```python
from build123d import *

# Parameters (mm, degrees)
SKETCH018_R          = 70
PAD010_DEPTH         = 7
SKETCH019_R          = 2.5
POCKET_DEPTH         = 3.5
POLARPATTERN_COUNT   = 4
SKETCH_R             = 7.5
SKETCH_R_2           = 5
PAD_DEPTH            = 20
SKETCH020_R          = 2.5
POCKET005_DEPTH      = 70.001
POCKET005_DEPTH_BACK = 70.001


with BuildPart() as part:
    # Sketch018 → Pad010 (new body)
    with BuildSketch(Plane.XY):
        Circle(SKETCH018_R)
    extrude(amount=PAD010_DEPTH)

    # Sketch019 → Pocket (cut)
    with BuildSketch(Plane.XY.offset(7)):
        with Locations((0, 60)):
            Circle(SKETCH019_R)
    pocket = extrude(amount=-POCKET_DEPTH, mode=Mode.SUBTRACT)

    # PolarPattern: Pocket ×4 about axis
    polarpattern_axis = Axis((0, 0, 7), (0, 0, 1))
    for i in range(1, POLARPATTERN_COUNT):
        add(pocket.rotate(polarpattern_axis, i * 360 / POLARPATTERN_COUNT), mode=Mode.SUBTRACT)

    # Sketch (on Face3 of PolarPattern) → Pad (join)
    with BuildSketch(Plane.XY.offset(7)):
        Circle(SKETCH_R)
        Circle(SKETCH_R_2, mode=Mode.SUBTRACT)
    extrude(amount=PAD_DEPTH)

    # Sketch020 → Pocket005 (cut, two sides)
    with BuildSketch(Plane.XZ) as pocket005_sk:
        with Locations((0, 20)):
            Circle(SKETCH020_R)
    extrude(amount=-POCKET005_DEPTH, mode=Mode.SUBTRACT)
    extrude(pocket005_sk.sketch, amount=POCKET005_DEPTH_BACK, mode=Mode.SUBTRACT)


solid = part.part
```
Verification items for the finished model (mm, model axes). A direction names the side the tool comes from. Give positions to 0.01 mm unless a question says otherwise; leave off trailing zeros. Order: outer loops, then holes, each group sorted by start corner. A loop starts at its lowest first (then second) coordinate and runs counter-clockwise, first axis right, second up. Notation, with made-up numbers: M 12.5,38 L 21.5,38 A32 cw 21.5,72 Z; hole C 62,3.5 d4. An arc over 180 degrees is marked long. Return JSON: item names as keys, results as strings. Group by question number.
1) Go/stop test with flat-tipped pins: pin 1 Ø6.5 at (x, y) = (60, 0) entering from +Z; pin 2 Ø8 at (x, z) = (0, 20) entering from +Y; pin 3 Ø2.5 at (x, y) = (59, -0.5) entering from +Z. Record where each tip stops, or that it passes through.
2) Section check D-D on x = 60. Record the cut outline in (y, z).
3) Scan lines: line 1 (Y direction, x = 0, z = 5.35); line 2 (Z direction, x = 8.5, y = -24); line 3 (X direction, y = -60, z = 5.75). Record each from-to range of solid material in increasing order.
4) Mould release check, pull along Z, two halves, no side actions. Record for faces 1 (the face through (2.385, 5.894, 20.751)), 2 (the face through (0.54, -57.56, 5.27)), 3 (the face through (60, 0, 3.5)): pulls with the +Z half, pulls with the -Z half, needs draft (parallel to the pull), parting line crosses it, or undercut.
5) Section check A-A on y = 0. Record the cut outline in (x, z), and give its area (4 significant figures).
6) Access from +Z, -Z, +X, -X, +Y, -Y to the whole of each face (thin tool, end or side, straight path). Record for faces 4 (the face through (2.385, -5.894, 20.751)), 5 (the face through (0, 60, 3.5)).
7) Section check B-B on x = 0. Record the cut outline in (y, z), and give its area (3 significant figures).
8) Section check C-C on z = 20. Record the cut outline in (x, y).
Answer block:
{
 "1": {"pin 1": "stops at z = 7", "pin 2": "stops at y = 7.5", "pin 3": "stops at z = 3.5"},
 "2": {"outline": "M -36.06,0 L 36.06,0 L 36.06,7 L 2.5,7 L 2.5,3.5 L -2.5,3.5 L -2.5,7 L -36.06,7 Z"},
 "3": {"line 1": "y = -70 to -62.5, -57.5 to 57.5, 62.5 to 70", "line 2": "z = 0 to 7", "line 3": "x = -36.06 to -2.5, 2.5 to 36.06"},
 "4": {"face 1": "undercut", "face 2": "needs draft", "face 3": "pulls with the +Z half"},
 "5": {"outline": "M -70,0 L 70,0 L 70,7 L 62.5,7 L 62.5,3.5 L 57.5,3.5 L 57.5,7 L 7.5,7 L 7.5,27 L 5,27 L 5,7 L -5,7 L -5,27 L -7.5,27 L -7.5,7 L -57.5,7 L -57.5,3.5 L -62.5,3.5 L -62.5,7 L -70,7 Z", "area": "1,045 mm^2"},
 "6": {"face 4": "+Y, -Y", "face 5": "+Z"},
 "7": {"outline": "M -70,0 L 70,0 L 70,7 L 62.5,7 L 62.5,3.5 L 57.5,3.5 L 57.5,7 L 7.5,7 L 7.5,17.5 L 5,17.5 L 5,7 L -5,7 L -5,17.5 L -7.5,17.5 L -7.5,7 L -57.5,7 L -57.5,3.5 L -62.5,3.5 L -62.5,7 L -70,7 Z; M -7.5,22.5 L -5,22.5 L -5,27 L -7.5,27 Z; M 5,22.5 L 7.5,22.5 L 7.5,27 L 5,27 Z", "area": "1,020 mm^2"},
 "8": {"outline": "M -2.5,-7.07 L -2.5,-4.33 A5 cw -2.5,4.33 L -2.5,7.07 A7.5 ccw Z; M 2.5,-7.07 A7.5 ccw 2.5,7.07 L 2.5,4.33 A5 cw 2.5,-4.33 Z"}
}
